Could you check a few things on this model? Use its own coordinates, in mm. Face numbers are marked on the shaded views. A direction names the side the tool comes from. Round coordinates to 2 decimals unless told otherwise and drop trailing zeros. Loops run counter-clockwise (first coordinate to the right, second up) from the corner with the lowest first, then second, coordinate; pieces in that order, holes last. Notation, with made-up numbers: (-10, 24.25) - (12, 24.25) arc R15 cw to (12, 33.25) - close; hole circle Ø5 at (75, -16.75). An arc over 180 degrees is marked (long way). Use one line per item in the form item = value.
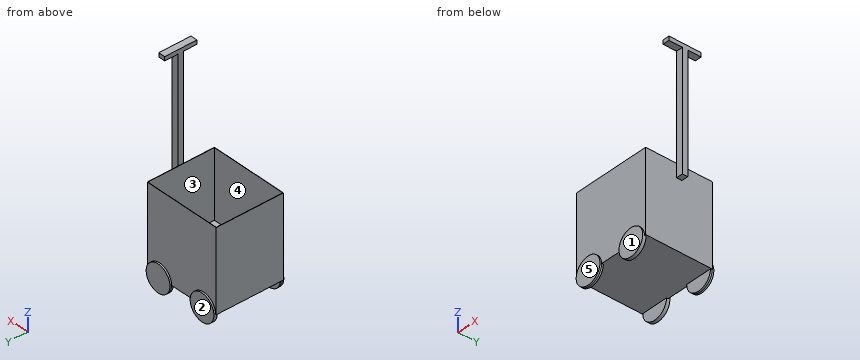
```python
from build123d import *

# Parameters (mm, degrees)
F0_W      = 580
F0_H      = 600
F1_DEPTH  = 500
F2_W      = 576
F2_H      = 496
F3_DEPTH  = 500
F4_W      = 40
F4_H      = 800
F4_H_2    = 100
F5_DEPTH  = 50
F6_W      = 50
F6_H      = 100
F7_DEPTH  = 30
F9_DEPTH  = 12.5
F11_DEPTH = 12.5


with BuildPart() as f1:
    # F0 (on Front) → F1 (new body)
    with BuildSketch(Plane.XZ):
        with Locations((1.860235, 108.586439)):
            Rectangle(F0_W, F0_H)
    extrude(amount=F1_DEPTH)

    # F2 (on face) → F3 (cut)
    with BuildSketch(Plane.XY.offset(408.586439)):
        with Locations((1.860235, -250)):
            Rectangle(F2_W, F2_H)
    extrude(amount=-F3_DEPTH, mode=Mode.SUBTRACT)

    # F4 (on face) → F5 (join)
    with BuildSketch(Plane.YZ.offset(291.860235)):
        with Locations((-250, 808.586439)):
            Rectangle(F4_W, F4_H)
        with Locations((-250, 358.586439)):
            Rectangle(F4_W, F4_H_2)
    extrude(amount=F5_DEPTH)

    # F6 (on face) → F7 (join)
    with BuildSketch(Plane.XY.offset(1208.586439)):
        with Locations((316.860235, -320)):
            Rectangle(F6_W, F6_H)
        with Locations((316.860235, -180)):
            Rectangle(F6_W, F6_H)
    extrude(amount=-F7_DEPTH)

    # F8 (on face) → F9 (join, symmetric)
    with BuildSketch(Plane.XZ.offset(500)):
        with BuildLine():
            Line((-278.139765, -191.413561), (-78.139765, -191.413561))
            ThreePointArc((-78.139765, -191.413561), (-178.139765, -91.413561), (-278.139765, -191.413561))
        make_face()
        with BuildLine():
            ThreePointArc((-278.139765, -191.413561), (-178.139765, -291.413561), (-78.139765, -191.413561))
            Line((-78.139765, -191.413561), (-278.139765, -191.413561))
        make_face()
        with BuildLine():
            Line((281.860235, -191.413561), (81.860235, -191.413561))
            ThreePointArc((81.860235, -191.413561), (181.860235, -291.413561), (281.860235, -191.413561))
        make_face()
        with BuildLine():
            ThreePointArc((281.860235, -191.413561), (181.860235, -91.413561), (81.860235, -191.413561))
            Line((81.860235, -191.413561), (281.860235, -191.413561))
        make_face()
    extrude(amount=F9_DEPTH, both=True)

    # F10 (on face) → F11 (join, symmetric)
    with BuildSketch(Plane(origin=(0, 0, 0), x_dir=(-1, 0, 0), z_dir=(0, 1, 0))):
        with BuildLine():
            Line((-286.860235, -191.413561), (-86.860235, -191.413561))
            ThreePointArc((-86.860235, -191.413561), (-186.860235, -91.413561), (-286.860235, -191.413561))
        make_face()
        with BuildLine():
            ThreePointArc((-286.860235, -191.413561), (-186.860235, -291.413561), (-86.860235, -191.413561))
            Line((-86.860235, -191.413561), (-286.860235, -191.413561))
        make_face()
        with BuildLine():
            Line((283.139765, -191.413561), (83.139765, -191.413561))
            ThreePointArc((83.139765, -191.413561), (183.139765, -291.413561), (283.139765, -191.413561))
        make_face()
        with BuildLine():
            ThreePointArc((283.139765, -191.413561), (183.139765, -91.413561), (83.139765, -191.413561))
            Line((83.139765, -191.413561), (283.139765, -191.413561))
        make_face()
    extrude(amount=F11_DEPTH, both=True)


solid = f1.part
```
1. Please list where these lines run through material, in increasing order: line 1 along X through (y, z) = (-23.5, 159.5); line 2 along Y through (x, z) = (118, 283); line 3 along Z through (x, y) = (43, -272).
Solution:
line_1 = -288.14 to -286.14, 289.86 to 291.86
line_2 = -500 to -498, -2 to 0
line_3 = -191.41 to -91.41
2. If we section it at A-A, the plane z = 12.5: Write out the boundary of the cut face in (x, y).
Solution:
outline = (-288.14, -500) - (291.86, -500) - (291.86, 0) - (-288.14, 0) - close; hole (-286.14, -498) - (289.86, -498) - (289.86, -2) - (-286.14, -2) - close
3. For P1, Ø24, axis at x = 320.5, z = 1191, coming from the -Y side; P2, Ø4, axis at x = 4, z = -29.5, coming from the +Y side; P3, Ø1.5, axis at x = -179, y = -344, coming from the +Z side, each with a flat end and sliding along its axis, tell me the tip position at first contact or that it passes through.
Solution:
P1 = -370
P2 = 0
P3 = -91.41
4. If we section it at B-B, the plane x = -5.5: Write out the boundary of the cut face in (y, z), plus the area to 3 significant figures.
Solution:
outline = (-500, -191.41) - (0, -191.41) - (0, 408.59) - (-2, 408.59) - (-2, -91.41) - (-498, -91.41) - (-498, 408.59) - (-500, 408.59) - close
area = 52,000 mm^2
5. If we section it at C-C, the plane y = -450: Write out the boundary of the cut face in (x, z).
Solution:
outline = (-288.14, -191.41) - (291.86, -191.41) - (291.86, 408.59) - (289.86, 408.59) - (289.86, -91.41) - (-286.14, -91.41) - (-286.14, 408.59) - (-288.14, 408.59) - close
6. If we section it at D-D, the plane y = -284.5: Write out the boundary of the cut face in (x, z), plus the area to 3 significant figures.
Solution:
outline = (-288.14, -191.41) - (291.86, -191.41) - (291.86, 408.59) - (289.86, 408.59) - (289.86, -91.41) - (-286.14, -91.41) - (-286.14, 408.59) - (-288.14, 408.59) - close; (291.86, 1178.59) - (341.86, 1178.59) - (341.86, 1208.59) - (291.86, 1208.59) - close
area = 61,500 mm^2
7. On a 3-axis mill with a long thin cutter (end or side, diameter ignored), from which of +Z, -Z, +X, -X, +Y, -Y can I reach the whole of each face in a straight line? I mean the marked faces 4 and 5. Say none if no direction works.
Solution:
face_4 = +Z
face_5 = +Z, -Z, +X, -X, -Y
8. We'd pull the mould along Y, two halves only. Please class the marked faces 1, 2 and 3: +Y half, -Y half, draft (parallel to the pull), parting line (faces both ways), or undercut.
Solution:
face_1 = -Y half
face_2 = +Y half
face_3 = undercut
